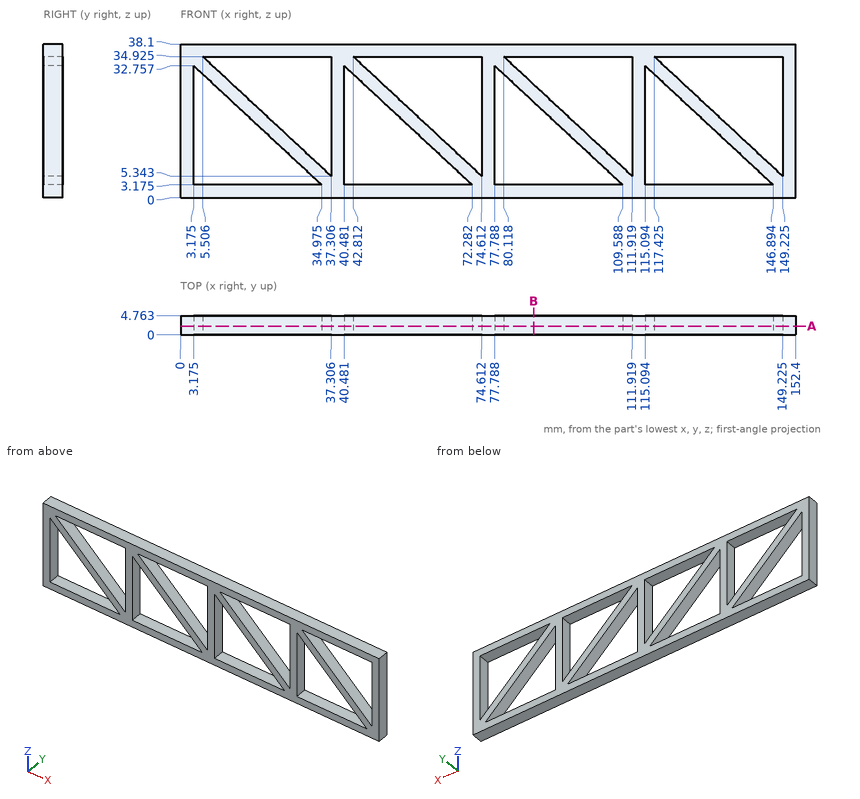
Input: dimensioned drawing with shaded views. Units: mm. Origin: part minimum x, y, z. Coordinates: 2 decimals unless noted, no trailing zeros. Order: outer loops, then holes, each group sorted by start corner. A loop starts at its lowest first (then second) coordinate and runs counter-clockwise, first axis right, second up.
1. Ray query, line 1 along Z through (x, y) = (119, 1.35) (1 decimal); line 2 along Z through (x, y) = (143, 1.35) (1 decimal); line 3 along Z through (x, y) = (115.5, 1.35) (1 decimal). Return the intervals inside material, ascending.
Checked values:
line 1: z = 0 to 3.2, 29.1 to 33.5, 34.9 to 38.1
line 2: z = 0 to 3.2, 6.8 to 11.1, 34.9 to 38.1
line 3: z = 0 to 3.2, 32.4 to 38.1
2. Cut plane B-B, the plane x = 87.5. Return loops of the section in (y, z) (1 decimal).
Checked values:
outline: (0, 0) - (4.8, 0) - (4.8, 3.2) - (0, 3.2) - close; (0, 23.7) - (4.8, 23.7) - (4.8, 28.1) - (0, 28.1) - close; (0, 34.9) - (4.8, 34.9) - (4.8, 38.1) - (0, 38.1) - close
3. Cut plane A-A, the plane y = 2.2. Count the separate pieces of the cut face and the enclosed holes in it, plus the area to 3 significant figures.
Checked values:
separate pieces: 1
enclosed holes: 8
area: 2,040 mm2
